Read the model definition and answer for the solid it produces. Units are mm, in the model's axes. A direction names the side the tool comes from. Coordinates: 2 decimals unless noted, no trailing zeros. Write each loop counter-clockwise with the first axis right and the second up, starting at its lowest first coordinate (ties: lowest second). Pieces come first, ordered by that corner, then holes.
1) Each of these flat-tipped pins is pushed along its axis until it touches: pin 1 Ø2.5 at (x, y) = (-19.53, 18.2) entering from +Z; pin 2 Ø3.5 at (x, y) = (-21.79, -13.63) entering from +Z. Where does it stop, or does it pass through?
2) Find the intervals of material crossed by line 1 (X direction, y = 18, z = -9.6); line 2 (Y direction, x = -7.5, z = -8.5); line 3 (Y direction, x = 2, z = -8.7), in increasing order.
3) Which of the six approach directions +Z, -Z, +X, -X, +Y, -Y give full straight-line access (tool end or side, diameter ignored) to faces 4 (the face through (3.36, 4, -9)), 5 (the face through (-7, -8, -8))?
4) The part is cut by section A-A (y = 5.5). Determine the outline of the cut face in (x, z).
5) The part is cut by section B-B (x = -2). Determine the outline of the cut face in (y, z), then the cut area to 3 significant figures.
6) Determine the mould class of faces 1 (the face through (-35.54, -9, -9)), 2 (the face through (-6, -46.997, -9)), 3 (the face through (-3, 9.203, -9)) for opening direction X: +X half, -X half, draft (parallel to the pull), parting line (faces both ways), or undercut.
7) The part is cut by section C-C (z = -8.55). Determine the outline of the cut face in (x, y), then the cut area to 3 significant figures.
from build123d import *

# Parameters (mm, degrees)
SKETCH1_W           = 57.9
SKETCH1_H           = 76.2
BOSS_EXTRUDE1_DEPTH = 2
SKETCH2_R           = 2
SKETCH2_W           = 12
SKETCH2_H           = 10
SKETCH2_R_2         = 1.5
CUT_EXTRUDE1_DEPTH  = 2
SKETCH4_R           = 2
SKETCH4_R_2         = 1.5
SKETCH4_R_3         = 1.957178151
BOSS_EXTRUDE5_DEPTH = 2
SKETCH8_W           = 57.9
SKETCH8_H           = 76.2
SKETCH8_R           = 2
SKETCH8_R_2         = 1.5
SKETCH8_W_2         = 12
SKETCH8_H_2         = 10
BOSS_EXTRUDE6_DEPTH = 10
SKETCH9_R           = 2
CUT_EXTRUDE6_DEPTH  = 10
SKETCH10_W          = 57.9
SKETCH10_H          = 76.2
CUT_EXTRUDE7_DEPTH  = 10


with BuildPart() as part:
    # Sketch1 → Boss-Extrude1 (new body)
    with BuildSketch(Plane.XY):
        with Locations((-6.590392234, -8.896581688)):
            Rectangle(SKETCH1_W, SKETCH1_H)
    extrude(amount=BOSS_EXTRUDE1_DEPTH)

    # Sketch2 → Cut-Extrude1 (cut)
    with BuildSketch(Plane(origin=(0, 0, 0), x_dir=(-1, 0, 0), z_dir=(0, 0, -1))):
        with Locations((-6.409607766, 14.203418312)):
            Circle(SKETCH2_R)
        with Locations((19.590392234, 14.203418312)):
            Circle(SKETCH2_R)
        with Locations((2.640392234, 4.203418312)):
            Rectangle(SKETCH2_W, SKETCH2_H)
        with Locations((16.590392234, -41.996581688)):
            Circle(SKETCH2_R)
        with Locations((-3.409607766, -41.996581688)):
            Circle(SKETCH2_R)
        with Locations((21.790392234, -13.626581688)):
            Circle(SKETCH2_R_2)
    extrude(amount=-CUT_EXTRUDE1_DEPTH, mode=Mode.SUBTRACT)

    # Sketch4 → Boss-Extrude5 (add)
    # profile 1 of 3: a face of its own
    with BuildSketch(Plane(origin=(0, 0, 0), x_dir=(-1, 0, 0), z_dir=(0, 0, -1))):
        Polygon((35.540392234, 29.203418312), (6.590392234, 29.203418312), (-22.359607766, 29.203418312), (-22.359607766, -46.996581688), (35.540392234, -46.996581688), align=None)
        with Locations((-3.409607766, -41.996581688)):
            Circle(SKETCH4_R, mode=Mode.SUBTRACT)
        with Locations((16.590392234, -41.996581688)):
            Circle(SKETCH4_R, mode=Mode.SUBTRACT)
        with Locations((21.790392234, -13.626581688)):
            Circle(SKETCH4_R_2, mode=Mode.SUBTRACT)
        Polygon((-13.650237399, 24.487372027), (6.590392234, 24.487372027), (30.150370064, 24.487372027), (30.150370064, 9.203418312), (8.640392234, 9.203418312), (8.640392234, -0.796581688), (-3.359607766, -0.796581688), (-3.359607766, 9.203418312), (-13.650237399, 9.203418312), align=None, mode=Mode.SUBTRACT)
    # profile 2 of 3: a face of its own
    with BuildSketch(Plane(origin=(0, 0, 0), x_dir=(-1, 0, 0), z_dir=(0, 0, -1))):
        with Locations((-6.409607766, 14.203418312)):
            Circle(SKETCH4_R)
    # profile 3 of 3: a face of its own
    with BuildSketch(Plane(origin=(0, 0, 0), x_dir=(-1, 0, 0), z_dir=(0, 0, -1))):
        with Locations((19.590392234, 14.203418312)):
            Circle(SKETCH4_R_3)
    extrude(amount=-BOSS_EXTRUDE5_DEPTH)


with BuildPart() as boss_extrude5_piece_1:
    # of the separate pieces the step leaves, piece 1, a body of its own (boss_extrude5_pieces)
    add(part.part.solids().sort_by_distance((-35.540392234, 29.203418312, 0))[0])



with BuildPart() as boss_extrude5_piece_2:
    # of the separate pieces the step leaves, piece 2, a body of its own (boss_extrude5_pieces)
    add(part.part.solids().sort_by_distance((-21.547570385, 14.203418312, 0))[0])


with BuildPart() as boss_extrude5_piece_1_1:
    add(boss_extrude5_piece_1.part)

    add(boss_extrude5_piece_2.part)  # Boss-Extrude6 merges Boss-Extrude5 piece 2
    # Sketch8 → Boss-Extrude6 (add)
    # profile 1 of 2: a face of its own
    with BuildSketch(Plane(origin=(0, 0, 0), x_dir=(-1, 0, 0), z_dir=(0, 0, -1))):
        with Locations((6.590392234, -8.896581688)):
            Rectangle(SKETCH8_W, SKETCH8_H)
        with Locations((16.590392234, -41.996581688)):
            Circle(SKETCH8_R, mode=Mode.SUBTRACT)
        with Locations((21.790392234, -13.626581688)):
            Circle(SKETCH8_R_2, mode=Mode.SUBTRACT)
        with Locations((19.590392234, 14.203418312)):
            Circle(SKETCH8_R, mode=Mode.SUBTRACT)
        with Locations((-3.409607766, -41.996581688)):
            Circle(SKETCH8_R, mode=Mode.SUBTRACT)
        with Locations((2.640392234, 4.203418312)):
            Rectangle(SKETCH8_W_2, SKETCH8_H_2, mode=Mode.SUBTRACT)
    # profile 2 of 2: a face of its own
    with BuildSketch(Plane(origin=(0, 0, 0), x_dir=(-1, 0, 0), z_dir=(0, 0, -1))):
        with Locations((19.590392234, 14.203418312)):
            Circle(SKETCH8_R)
    extrude(amount=BOSS_EXTRUDE6_DEPTH)

    # Sketch9 → Cut-Extrude6 (cut)
    with BuildSketch(Plane(origin=(0, 0, -10), x_dir=(-1, 0, 0), z_dir=(0, 0, -1))):
        with Locations((-6.468155069, 18.203418312)):
            Circle(SKETCH9_R)
        with Locations((19.531844931, 18.203418312)):
            Circle(SKETCH9_R)
    extrude(amount=-CUT_EXTRUDE6_DEPTH, mode=Mode.SUBTRACT)

    # Sketch10 → Cut-Extrude7 (cut)
    with BuildSketch(Plane.XY.offset(2)):
        with Locations((-6.590392234, -8.896581688)):
            Rectangle(SKETCH10_W, SKETCH10_H)
    extrude(amount=-CUT_EXTRUDE7_DEPTH, mode=Mode.SUBTRACT)


solid = boss_extrude5_piece_1_1.part
Reported:
1. pin 1: passes through
1. pin 2: stops at z = -8
2. line 1: x = -35.54 to -21.52, -17.54 to 4.48, 8.46 to 22.36
2. line 2: y = -47 to -0.8, 9.2 to 29.2
2. line 3: y = -47 to -43.42, -40.58 to -0.8, 9.2 to 29.2
3. face 4: +Z, -Z
3. face 5: +Z, +X, -X, +Y, -Y
4. outline: (-35.54, -10) - (-8.64, -10) - (-8.64, -8) - (-35.54, -8) - close; (3.36, -10) - (22.36, -10) - (22.36, -8) - (3.36, -8) - close
5. outline: (-47, -10) - (-0.8, -10) - (-0.8, -8) - (-47, -8) - close; (9.2, -10) - (29.2, -10) - (29.2, -8) - (9.2, -8) - close
5. area: 132 mm2
6. face 1: -X half
6. face 2: draft
6. face 3: undercut
7. outline: (-35.54, -47) - (22.36, -47) - (22.36, 29.2) - (-35.54, 29.2) - close; hole circle Ø3 at (-21.79, -13.63); hole circle Ø4 at (-19.53, 18.2); hole circle Ø4 at (-16.59, -42); hole (-8.64, -0.8) - (3.36, -0.8) - (3.36, 9.2) - (-8.64, 9.2) - close; hole circle Ø4 at (3.41, -42); hole circle Ø4 at (6.47, 18.2)
7. area: 4,230 mm2
